Check sheet for the modelled part. Datum: model origin and axes. Units: mm. A direction names the side the tool comes from. Give positions to 0.01 mm unless a question says otherwise; leave off trailing zeros. Loops run counter-clockwise (first coordinate to the right, second up) from the corner with the lowest first, then second, coordinate; pieces in that order, holes last. Notation, with made-up numbers: M -2.75,36 L 1.25,36 A28 cw 1.25,63 Z; hole C -29.75,-35.75 d6. An arc over 180 degrees is marked long. Use one line per item in the form item = value.
Autodesk Inventor part; units mm, degrees
ref_plane "YZ Plane" through (0, 0, 0) normal (1, 0, 0) x (0, 1, 0)
ref_plane "XZ Plane" through (0, 0, 0) normal (0, 1, 0) x (-1, 0, 0)
ref_plane "XY Plane" through (0, 0, 0) normal (0, 0, 1) x (1, 0, 0)
sketch "Sketch1" plane through (0, 0, 0) normal (0, 1, 0) x (-1, 0, 0)
  circle A0 centre (0, 0) radius 12.7
  circle A1 centre (0, 0) radius 12.065
  dimension "d0" = 25.4
  dimension "d1" = 24.13
extrude "Extrusion1" add sketch "Sketch1" along normal blind 254
sketch "Sketch2" plane through (0, 0, 0) normal (0, -1, 0) x (1, 0, 0)
  circle A0 centre (0, 0) radius 12.065
  circle A1 centre (0, 0) radius 12.065
  circle A2 centre (0, 0) radius 6.35
  dimension "d4" = 12.7
extrude "Extrusion2" add sketch "Sketch2" against normal blind 1.27
sketch "Sketch3" plane through (0, 1.27, 0) normal (0, 1, 0) x (1, 0, 0)
  circle A0 centre (0, 0) radius 6.35
  circle A1 centre (0, 0) radius 5.588
  dimension "d7" = 12.7
  dimension "d8" = 11.176
extrude "Extrusion3" add sketch "Sketch3" against normal blind 50.8
properties part number "1in ss pipe" material "Stainless Steel"
1) Set-up check for faces 5 (the face through (-4.434, -23.774, 3.4)), 6 (the face through (-3, 0, 6)): record each of +Z, -Z, +X, -X, +Y, -Y from which the full face is reachable in a straight line by a thin tool's end or side.
Evaluation:
face_5 = +Y, -Y
face_6 = -Y
2) Section check A-A (z = 0). Record the cut outline in (x, y) (3 decimals).
Evaluation:
outline = M -12.7,0 L -6.35,0 L -6.35,-49.53 L -5.588,-49.53 L -5.588,1.27 L -12.065,1.27 L -12.065,254 L -12.7,254 Z; M 5.588,-49.53 L 6.35,-49.53 L 6.35,0 L 12.7,0 L 12.7,254 L 12.065,254 L 12.065,1.27 L 5.588,1.27 Z
3) Section check C-C (y = 106.5). Record the cut outline in (x, z) (3 decimals), then the cut area to 3 significant figures.
Evaluation:
outline = C 0,0 d25.4; hole C 0,0 d24.13
area = 49.4 mm^2
4) Section check B-B (x = 0). Record the cut outline in (y, z) (3 decimals), then the cut area to 3 significant figures.
Evaluation:
outline = M -49.53,-6.35 L 0,-6.35 L 0,-12.7 L 254,-12.7 L 254,-12.065 L 1.27,-12.065 L 1.27,-5.588 L -49.53,-5.588 Z; M -49.53,5.588 L 1.27,5.588 L 1.27,12.065 L 254,12.065 L 254,12.7 L 0,12.7 L 0,6.35 L -49.53,6.35 Z
area = 415 mm^2
5) Scan lines: line 1 (X direction, y = -15, z = 0); line 2 (Z direction, x = 0, y = 202.5) (3 decimals). Record each from-to range of solid material in increasing order.
Evaluation:
line_1 = -6.35 to -5.59, 5.59 to 6.35
line_2 = -12.7 to -12.065, 12.065 to 12.7
6) Depth check by flat-ended pin: pin 1 Ø6 at (x, z) = (8, 2.5) entering from +Y; pin 2 Ø1.5 at (y, z) = (214, 2) entering from +X; pin 3 Ø1 at (x, y) = (6.5, 17) entering from -Z; pin 4 Ø4 at (x, z) = (10, 10) entering from +Y. Enter the tip coordinate at first touch or a pass-through.
Evaluation:
pin_1 = 1.27
pin_2 = 12.64
pin_3 = -11.19
pin_4 = 254
7) Release check for a two-part mould opening along Z. For faces 1 (the face through (0, -49.53, 6)), 2 (the face through (-1.38, -24.42, 6.2)), 3 (the face through (5, 1.27, 3)), 4 (the face through (-11.51, 125.87, -3.62)) record: pulls with the +Z half, pulls with the -Z half, needs draft (parallel to the pull), parting line crosses it, or undercut.
Evaluation:
face_1 = needs draft
face_2 = parting line crosses it
face_3 = undercut
face_4 = undercut
8) Section check D-D (y = -7.5). Record the cut outline in (x, z), then the cut area to 3 significant figures.
Evaluation:
outline = C 0,0 d12.7; hole C 0,0 d11.18
area = 28.6 mm^2
